from build123d import *

# Parameters (mm, degrees)
F0_W     = 450
F0_H     = 450
F1_DEPTH = 950
F2_W     = 66.2090092897
F2_H     = 425
F2_W_2   = 313.7909907103
F2_H_2   = 50
F3_DEPTH = 450.001
F4_W     = 380
F4_H     = 425
F5_DEPTH = 450.001
F6_W     = 380
F6_H     = 50
F6_H_2   = 304.5921526788
F7_DEPTH = 165.8159708686


with BuildPart() as f1:
    # F0 (on Top) → F1 (new body)
    with BuildSketch(Plane.XY):
        Rectangle(F0_W, F0_H)
    extrude(amount=F1_DEPTH)

    # F2 (on face) → F3 (cut, through all)
    with BuildSketch(Plane.XZ.offset(225)):
        Polygon((-225, 475), (123.7909907103, 475), (190, 950), (-225, 950), align=None)
        Polygon((158.7909907103, 475), (225, 475), (225, 950), align=None)
        with Locations((191.8954953551, 212.5)):
            Rectangle(F2_W, F2_H)
        with Locations((-33.1045046449, 212.5)):
            Rectangle(F2_W_2, F2_H)
        with Locations((191.8954953551, 450)):
            Rectangle(F2_W, F2_H_2)
    extrude(amount=-F3_DEPTH, mode=Mode.SUBTRACT)

    # F4 (on face) → F5 (cut, through all)
    with BuildSketch(Plane(origin=(-225, 0, 0), x_dir=(0, -1, 0), z_dir=(-1, 0, 0))):
        with Locations((0, 212.5)):
            Rectangle(F4_W, F4_H)
    extrude(amount=-F5_DEPTH, mode=Mode.SUBTRACT)

    # F6 (on face) → F7 (cut, through all)
    with BuildSketch(Plane(origin=(56.4845518778, 0, -7.8732341474), x_dir=(0, -1, 0), z_dir=(-0.9904248794, 0, 0.1380527369))):
        with Locations((0, 867.1336554909)):
            Rectangle(F6_W, F6_H)
        with Locations((0, 639.8375791515)):
            Rectangle(F6_W, F6_H_2)
    extrude(amount=-F7_DEPTH, mode=Mode.SUBTRACT)


solid = f1.part
Can you work these out from the model? Positions are in its coordinate system, mm. A direction names the side the tool comes from. Round coordinates to 2 decimals unless told otherwise and drop trailing zeros. Loops run counter-clockwise (first coordinate to the right, second up) from the corner with the lowest first, then second, coordinate; pieces in that order, holes last. Notation, with made-up numbers: (-36, 29) - (6, 29) arc R11 ccw to (6, 43) - close; hole circle Ø10 at (-23.5, 21.25). An arc over 180 degrees is marked (long way). Write item = value, one per line. Start each with the question number.
(1) If we section it at A-A (z = 285): Please give me the cut outline in (x, y), and give its area (3 significant figures).
(2) If we mould it in two halves opening along Z, with no side actions, what happens to faces 4 (the face through (141, 190, 210)), 5 (the face through (141, 2.7, 472.6)), 6 (the face through (193, -190, 848))? For each: released by +Z, released by -Z, zero draft, split by the parting line, or undercut.
(3) If we section it at B-B (y = -61): Please give me the cut outline in (x, z).
(4) If we section it at D-D (x = -20.5): Please give me the cut outline in (y, z).
(5) If I drill on probe 1 along Y at (x, z) = (169.5, 666); probe 2 along Z at (x, y) = (116, -139.5); probe 3 along X at (y, z) = (191, 273.5), over which ranges is the centre line in solid material (lowest first)? Write a range as [from, to].
(6) If we section it at C-C (z = 704.5): Please give me the cut outline in (x, y), and give its area (3 significant figures).
(7) For P1, Ø10, axis at x = -64.5, y = -163, coming from the -Z side; P2, Ø4, axis at x = -118, y = -106.5, coming from the +Z side; P3, Ø4, axis at y = -6, z = 441, coming from the +X side, each with a flat end and sliding along its axis, tell me the tip position at first contact or that it passes through.
(8) For faces 1 (the face through (158.791, -1, 432)), 2 (the face through (123.791, -208, 210)), 3 (the face through (-208, -190, 210)), which set-ups out of +Z, -Z, +X, -X, +Y, -Y let a thin tool reach every point of the face, with its end or its side?
Ans:
q1.outline = (-225, -225) - (-190, -225) - (-190, -190) - (-225, -190) - close; (-225, 190) - (-190, 190) - (-190, 225) - (-225, 225) - close; (123.79, -225) - (158.79, -225) - (158.79, -190) - (123.79, -190) - close; (123.79, 190) - (158.79, 190) - (158.79, 225) - (123.79, 225) - close
q1.area = 4,900 mm²
q2.face_4 = zero draft
q2.face_5 = released by +Z
q2.face_6 = undercut
q3.outline = (-225, 425) - (158.79, 425) - (158.79, 470.12) - (123.79, 475) - (-225, 475) - close; (165.84, 776.68) - (200.17, 771.89) - (207.08, 821.41) - (172.74, 826.2) - close; (179.65, 875.72) - (213.98, 870.93) - (225, 950) - (190, 950) - close
q4.outline = (-225, 425) - (225, 425) - (225, 475) - (-225, 475) - close
q5.probe_1 = [-225, -190], [190, 225]
q5.probe_2 = [425, 475]
q5.probe_3 = [-225, -190], [123.79, 158.79]
q6.outline = (155.78, -225) - (190.78, -225) - (190.78, -190) - (155.78, -190) - close; (155.78, 190) - (190.78, 190) - (190.78, 225) - (155.78, 225) - close
q6.area = 2,450 mm²
q7.P1 = 425
q7.P2 = 475
q7.P3 = 158.79
q8.face_1 = -Z, +X, +Y, -Y
q8.face_2 = -Z, +Y, -Y
q8.face_3 = -Z, +X, -X
